```python
from build123d import *

# Parameters (mm, degrees)
F0_R     = 10
F1_DEPTH = 3
F2_W     = 10
F2_H     = 10
F3_DEPTH = 3.001


with BuildPart() as f1:
    # F0 (on Top) → F1 (new body)
    with BuildSketch(Plane.XY):
        Circle(F0_R)
    extrude(amount=F1_DEPTH)

    # F2 (on face) → F3 (cut, through all)
    with BuildSketch(Plane.XY.offset(3)):
        Rectangle(F2_W, F2_H)
    extrude(amount=-F3_DEPTH, mode=Mode.SUBTRACT)


solid = f1.part
```
Geometry: final body of the model. Coordinates: model frame, mm. A direction names the side the tool comes from. Coordinates: 2 decimals unless noted, no trailing zeros. Order: outer loops, then holes, each group sorted by start corner. A loop starts at its lowest first (then second) coordinate and runs counter-clockwise, first axis right, second up. Notation, with made-up numbers: M -23.5,73.5 L -9.5,73.5 A24 cw -9.5,101.5 Z; hole C 26.5,-18 d9. An arc over 180 degrees is marked long. Answer in a Markdown table with one row per item. Add a question column.
Q1. Section query D-D on y = 8. Return the cut outline in (x, z), and give its area (3 significant figures).
Q2. Section query C-C on z = 2.7. Return the cut outline in (x, y), and give its area (3 significant figures).
Q3. Reachability of faces 5 (the flat face through (5, 0, 2)), 6 (the flat face through (7, 0, 3)) from +Z, -Z, +X, -X, +Y, -Y: full face, straight path, thin tool, end or side. Return the list, or none.
Q4. Contact query for flat-ended pins moving along their axis: P1, Ø0.9, axis at x = -1, z = 2, coming from the +Y side; P2, Ø1, axis at y = -5.5, z = 1, coming from the +X side; P3, Ø1.5, axis at y = -1.5, z = 1, coming from the +X side. Output: stop coordinate, or through.
Q5. Mould query, pull axis X, two halves, no side actions, for faces 1 (the flat face through (7, 0, 0)), 2 (the flat face through (0, -5, 2)), 3 (the cylindrical face through (-2.17, -9.76, 1.48)), 4 (the flat face through (0, 5, 2)). Classes: released by +X, released by -X, zero draft, split by the parting line, or undercut.
Q6. Line query: L1, parallel to X at y = 0.25, z = 1.3; L2, parallel to Y at x = -4.25, z = 1; L3, parallel to Y at x = 4.5, z = 2.3. Output: solid intervals per line, ascending.
Q7. Section query A-A on x = 0. Return the cut outline in (y, z), and give its area (3 significant figures).
Completed:
| question | item | result |
|---|---|---|
| 1 | outline | M -6,0 L 6,0 L 6,3 L -6,3 Z |
| 1 | area | 36.0 mm2 |
| 2 | outline | C 0,0 d20; hole M -5,-5 L 5,-5 L 5,5 L -5,5 Z |
| 2 | area | 214 mm2 |
| 3 | face 5 | +Z, -Z |
| 3 | face 6 | +Z, +X, -X, +Y, -Y |
| 4 | P1 | stops at y = 9.98 |
| 4 | P2 | stops at x = 8.66 |
| 4 | P3 | stops at x = 9.97 |
| 5 | face 1 | zero draft |
| 5 | face 2 | undercut |
| 5 | face 3 | split by the parting line |
| 5 | face 4 | undercut |
| 6 | L1 | x = -10 to -5, 5 to 10 |
| 6 | L2 | y = -9.05 to -5, 5 to 9.05 |
| 6 | L3 | y = -8.93 to -5, 5 to 8.93 |
| 7 | outline | M -10,0 L -5,0 L -5,3 L -10,3 Z; M 5,0 L 10,0 L 10,3 L 5,3 Z |
| 7 | area | 30.0 mm2 |
